Build history of the part. All positions in model axes, mm. A direction names the side the tool comes from. Give positions to 0.01 mm unless a question says otherwise; leave off trailing zeros. Order: outer loops, then holes, each group sorted by start corner. A loop starts at its lowest first (then second) coordinate and runs counter-clockwise, first axis right, second up. Notation, with made-up numbers: M 48,61.5 L 55,61.5 A26 ccw 55,88.5 Z; hole C 0,14 d3. An arc over 180 degrees is marked long. Answer as CSV lines item,"result".
from build123d import *

# Parameters (mm, degrees)
SKETCH1_W                      = 44
SKETCH1_H                      = 34
SKETCH1_R                      = 9
SKETCH1_R_2                    = 1.5
BASE_FLANGE1_DEPTH             = 2
EDGE_FLANGE1_STRIP_W           = 9.4732
EDGE_FLANGE1_STRIP_H           = 2
EDGE_FLANGE1_STRIP_CUT_DEPTH   = 34
EDGE_FLANGE1_STRIP_2_W         = 9.4732
EDGE_FLANGE1_STRIP_2_H         = 2
EDGE_FLANGE1_STRIP_CUT_2_DEPTH = 34
EDGE_FLANGE1_DEPTH             = 34
EDGE_FLANGE1_BEND_DEPTH        = 34
EDGE_FLANGE2_STRIP_W           = 9.4732
EDGE_FLANGE2_STRIP_H           = 2
EDGE_FLANGE2_STRIP_CUT_DEPTH   = 34
EDGE_FLANGE2_STRIP_2_W         = 9.4732
EDGE_FLANGE2_STRIP_2_H         = 2
EDGE_FLANGE2_STRIP_CUT_2_DEPTH = 34
EDGE_FLANGE2_DEPTH             = 34
EDGE_FLANGE2_BEND_DEPTH        = 34
SKETCH18_R                     = 3
CUT_EXTRUDE1_DEPTH             = 10


# Sheet-metal steps are written as plain solids
with BuildPart() as part:
    # Sketch1 → Base-Flange1 (new body)
    with BuildSketch(Plane.XY):
        Rectangle(SKETCH1_W, SKETCH1_H)
        Circle(SKETCH1_R, mode=Mode.SUBTRACT)
        with Locations((0, 13)):
            Circle(SKETCH1_R_2, mode=Mode.SUBTRACT)
        with Locations((13, 0)):
            Circle(SKETCH1_R_2, mode=Mode.SUBTRACT)
        with Locations((0, -13)):
            Circle(SKETCH1_R_2, mode=Mode.SUBTRACT)
        with Locations((-13, 0)):
            Circle(SKETCH1_R_2, mode=Mode.SUBTRACT)
    extrude(amount=-BASE_FLANGE1_DEPTH)

    # Edge-Flange1 strip (across the edge) → Edge-Flange1 strip cut (cut)
    with BuildSketch(Plane(origin=(-22, 17, 0), x_dir=(1, 0, 0), z_dir=(0, -1, 0))):
        with Locations((-4, -1)):
            Rectangle(EDGE_FLANGE1_STRIP_W, EDGE_FLANGE1_STRIP_H)
    extrude(amount=EDGE_FLANGE1_STRIP_CUT_DEPTH, mode=Mode.SUBTRACT)

    # Edge-Flange1 strip 2 (across the edge) → Edge-Flange1 strip cut 2 (cut)
    with BuildSketch(Plane(origin=(22, -17, 0), x_dir=(-1, 0, 0), z_dir=(0, 1, 0))):
        with Locations((-4, -1)):
            Rectangle(EDGE_FLANGE1_STRIP_2_W, EDGE_FLANGE1_STRIP_2_H)
    extrude(amount=EDGE_FLANGE1_STRIP_CUT_2_DEPTH, mode=Mode.SUBTRACT)

    # Edge-Flange1 section (across the edge) → Edge-Flange1 (add)
    with BuildSketch(Plane(origin=(-22, 17, 0), x_dir=(1, 0, 0), z_dir=(0, -1, 0))):
        with BuildLine():
            Line((-2, 0.7366), (-2, 11))
            Line((-2, 11), (0, 11))
            Line((0, 11), (0, 0.7366))
            ThreePointArc((0, 0.7366), (0.215745145, 0.215745145), (0.7366, 0))
            Line((0.7366, 0), (0.7366, -2))
            ThreePointArc((0.7366, -2), (-1.198468417, -1.198468417), (-2, 0.7366))
        make_face()
    extrude(amount=EDGE_FLANGE1_DEPTH)

    # Edge-Flange1 section 2 (across the edge) → Edge-Flange1 bend (add)
    with BuildSketch(Plane(origin=(22, -17, 0), x_dir=(-1, 0, 0), z_dir=(0, 1, 0))):
        with BuildLine():
            Line((-2, 0.7366), (-2, 11))
            Line((-2, 11), (0, 11))
            Line((0, 11), (0, 0.7366))
            ThreePointArc((0, 0.7366), (0.215745145, 0.215745145), (0.7366, 0))
            Line((0.7366, 0), (0.7366, -2))
            ThreePointArc((0.7366, -2), (-1.198468417, -1.198468417), (-2, 0.7366))
        make_face()
    extrude(amount=EDGE_FLANGE1_BEND_DEPTH)

    # Edge-Flange2 strip (across the edge) → Edge-Flange2 strip cut (cut)
    with BuildSketch(Plane(origin=(-24, -17, 11), x_dir=(0, 0, -1), z_dir=(0, 1, 0))):
        with Locations((-4, -1)):
            Rectangle(EDGE_FLANGE2_STRIP_W, EDGE_FLANGE2_STRIP_H)
    extrude(amount=EDGE_FLANGE2_STRIP_CUT_DEPTH, mode=Mode.SUBTRACT)

    # Edge-Flange2 strip 2 (across the edge) → Edge-Flange2 strip cut 2 (cut)
    with BuildSketch(Plane(origin=(24, 17, 11), x_dir=(0, 0, -1), z_dir=(0, -1, 0))):
        with Locations((-4, -1)):
            Rectangle(EDGE_FLANGE2_STRIP_2_W, EDGE_FLANGE2_STRIP_2_H)
    extrude(amount=EDGE_FLANGE2_STRIP_CUT_2_DEPTH, mode=Mode.SUBTRACT)

    # Edge-Flange2 section (across the edge) → Edge-Flange2 (add)
    with BuildSketch(Plane(origin=(-24, -17, 11), x_dir=(0, 0, -1), z_dir=(0, 1, 0))):
        with BuildLine():
            Line((-2, 0.7366), (-2, 41))
            Line((-2, 41), (0, 41))
            Line((0, 41), (0, 0.7366))
            ThreePointArc((0, 0.7366), (0.215745145, 0.215745145), (0.7366, 0))
            Line((0.7366, 0), (0.7366, -2))
            ThreePointArc((0.7366, -2), (-1.198468417, -1.198468417), (-2, 0.7366))
        make_face()
    extrude(amount=EDGE_FLANGE2_DEPTH)

    # Edge-Flange2 section 2 (across the edge) → Edge-Flange2 bend (add)
    with BuildSketch(Plane(origin=(24, 17, 11), x_dir=(0, 0, -1), z_dir=(0, -1, 0))):
        with BuildLine():
            Line((-2, 0.7366), (-2, 41))
            Line((-2, 41), (0, 41))
            Line((0, 41), (0, 0.7366))
            ThreePointArc((0, 0.7366), (0.215745145, 0.215745145), (0.7366, 0))
            Line((0.7366, 0), (0.7366, -2))
            ThreePointArc((0.7366, -2), (-1.198468417, -1.198468417), (-2, 0.7366))
        make_face()
    extrude(amount=EDGE_FLANGE2_BEND_DEPTH)

    # Sketch18 → Cut-Extrude1 (cut)
    with BuildSketch(Plane(origin=(0, 0, 11), x_dir=(-1, 0, 0), z_dir=(0, 0, -1))):
        with Locations((60, 0)):
            Circle(SKETCH18_R)
        with Locations((42, 0)):
            Circle(SKETCH18_R)
        with Locations((-60, 0)):
            Circle(SKETCH18_R)
        with Locations((-42, 0)):
            Circle(SKETCH18_R)
    extrude(amount=-CUT_EXTRUDE1_DEPTH, mode=Mode.SUBTRACT)


solid = part.part
Item 1: Band-saw the part on D-D (x = 0). Give the cut face in (y, z).
Geometry says:
outline,"M -17,-2 L -14.5,-2 L -14.5,0 L -17,0 Z; M -11.5,-2 L -9,-2 L -9,0 L -11.5,0 Z; M 9,-2 L 11.5,-2 L 11.5,0 L 9,0 Z; M 14.5,-2 L 17,-2 L 17,0 L 14.5,0 Z"
Item 2: Drop flat-ended pins along their axis: pin 1 (3 mm diameter, centred on x = -30.5, y = -1.5, fed in from -Z); pin 2 (3 mm diameter, centred on y = -5.5, z = 7.5, fed in from +X); pin 3 (17 mm diameter, centred on x = 1, y = 1.5, fed in from +Z); pin 4 (1.5 mm diameter, centred on x = -26, z = 6, fed in from -Y). Give the stop position or say it passes through.
Geometry says:
pin 1,"stops at z = 11"
pin 2,"stops at x = 24"
pin 3,"stops at z = 0"
pin 4,"passes through"
Item 3: Probe line 1 along Y through (x, z) = (0, -1.05); line 2 along Y through (x, z) = (13, -0.6); line 3 along X through (y, z) = (8, 3.75). List the from-to ranges inside material, lowest first. Write a range as from..to.
Geometry says:
line 1,"y = -17..-14.5, -11.5..-9, 9..11.5, 14.5..17"
line 2,"y = -17..-1.5, 1.5..17"
line 3,"x = -24..-22, 22..24"
Item 4: Pull direction Y, two halves, no side cores. Call faces 1 (the cylindrical face through (-39, 0, 12)), 2 (the flat face through (45, 4, 13)), 3 (the cylindrical face through (45, 0, 12)), 4 (the flat face through (-5, -17, -1)): released by +Y, released by -Y, zero draft, split by the parting line, or undercut.
Geometry says:
face 1,"undercut"
face 2,"zero draft"
face 3,"undercut"
face 4,"released by -Y"
Item 5: Band-saw the part on B-B (x = -13). Give the cut face in (y, z).
Geometry says:
outline,"M -17,-2 L -1.5,-2 L -1.5,0 L -17,0 Z; M 1.5,-2 L 17,-2 L 17,0 L 1.5,0 Z"
Item 6: Band-saw the part on C-C (y = 13). Give the cut face in (x, z).
Geometry says:
outline,"M -65,11 L -24.74,11 A0.74 cw -24,10.26 L -24,0.74 A2.74 ccw -21.26,-2 L -1.5,-2 L -1.5,0 L -21.26,0 A0.74 cw -22,0.74 L -22,10.26 A2.74 ccw -24.74,13 L -65,13 Z; M 1.5,-2 L 21.26,-2 A2.74 ccw 24,0.74 L 24,10.26 A0.74 cw 24.74,11 L 65,11 L 65,13 L 24.74,13 A2.74 ccw 22,10.26 L 22,0.74 A0.74 cw 21.26,0 L 1.5,0 Z"
Item 7: 3-axis set-ups, long thin cutter, end or side, ignore diameter. For faces 5 (the flat face through (-22, 0, 6)), 6 (the cylindrical face through (-1.172, 8.923, -0.986)), 7 (the flat face through (-45.2, -0.2, 11)), 8 (the flat face through (24, 0, 5)): which of +Z, -Z, +X, -X, +Y, -Y reach the whole face in a straight line?
Geometry says:
face 5,"+Z, +Y, -Y"
face 6,"+Z, -Z"
face 7,"-Z, -X, +Y, -Y"
face 8,"-Z, +X, +Y, -Y"
Item 8: Band-saw the part on A-A (z = 4). Give the cut face in (x, y).
Geometry says:
outline,"M -24,-17 L -22,-17 L -22,17 L -24,17 Z; M 22,-17 L 24,-17 L 24,17 L 22,17 Z"
